Read the model definition and answer for the solid it produces. Units are mm, in the model's axes. Face numbers are marked on the shaded views. A direction names the side the tool comes from. Coordinates: 2 decimals unless noted, no trailing zeros. Write each loop counter-clockwise with the first axis right and the second up, starting at its lowest first coordinate (ties: lowest second). Pieces come first, ordered by that corner, then holes. Notation, with made-up numbers: (-8.75, -11.75) -> (18.25, -11.75) arc R20 ccw to (18.25, 10.25) -> close; hole circle Ø10 at (-30.5, 88.25). An arc over 180 degrees is marked (long way). Use CSV: the item, a comma, the result in double quotes.
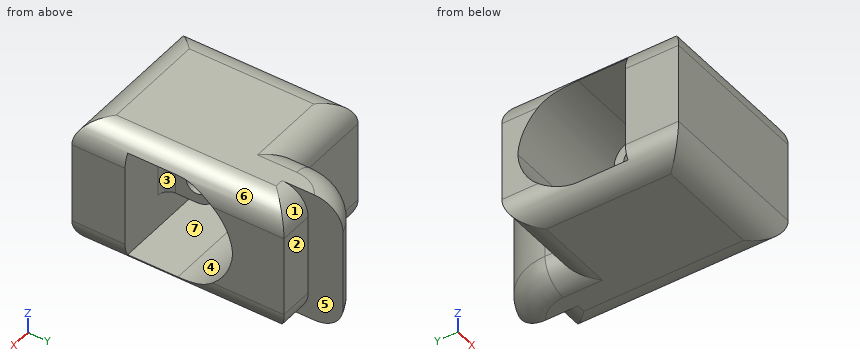
from build123d import *

# Parameters (mm, degrees)
BOSS_EXTRUDE1_DEPTH = 63.5
SKETCH3_W           = 103
SKETCH3_H           = 103
CUT_EXTRUDE1_DEPTH  = 211.692895559
BOSS_EXTRUDE2_DEPTH = 20
FILLET1_R           = 55
SKETCH6_R           = 10
CUT_EXTRUDE2_DEPTH  = 176.866755526
FILLET2_R           = 10
FILLET3_R           = 25


with BuildPart() as part:
    # Sketch2 → Boss-Extrude1 (new, symmetric)
    with BuildSketch(Plane.XY):
        with BuildLine():
            Line((-37.021158778, -102.394460884), (112.91726901, -102.394460884))
            Line((112.91726901, -102.394460884), (112.91726901, 63.318112544))
            Line((112.91726901, 63.318112544), (112.91726901, 100.457569387))
            Line((112.91726901, 100.457569387), (79.814777063, 100.457569387))
            Line((79.814777063, 100.457569387), (79.814777063, 133.707569387))
            ThreePointArc((79.814777063, 133.707569387), (50.885133933, 112.867809308), (39.821527553, 78.973614146))
            Line((39.821527553, 78.973614146), (39.821527553, 66.568112544))
            Line((39.821527553, 66.568112544), (-37.021158778, 66.568112544))
            Line((-37.021158778, 66.568112544), (-37.021158778, -102.394460884))
        make_face()
    extrude(amount=BOSS_EXTRUDE1_DEPTH, both=True)

    # Sketch3 → Cut-Extrude1 (cut, through all)
    with BuildSketch(Plane(origin=(112.91726901, 0, 0), x_dir=(0, 0, -1), z_dir=(1, 0, 0))):
        Rectangle(SKETCH3_W, SKETCH3_H)
    extrude(amount=-CUT_EXTRUDE1_DEPTH, mode=Mode.SUBTRACT)

    # Sketch5 → Boss-Extrude2 (add, symmetric)
    with BuildSketch(Plane.ZY.offset(-37.948055116)):
        with BuildLine():
            Line((19, -51.5), (-19, -51.5))
            Line((-19, -51.5), (-19, -21.5))
            ThreePointArc((-19, -21.5), (0, -2.5), (19, -21.5))
            Line((19, -21.5), (19, -51.5))
        make_face()
    extrude(amount=BOSS_EXTRUDE2_DEPTH, both=True)

    # Fillet1
    # the kernel refuses this fillet: 55 mm, written as the material it adds along each edge
    with BuildSketch(Plane(origin=(112.91726901, 51.5, 51.5), x_dir=(0, 0, -1), z_dir=(-1, 0, 0))) as fillet1_piece_1:
        with BuildLine():
            CenterArc((FILLET1_R, FILLET1_R), FILLET1_R, 180, 90)
            Line((0, FILLET1_R), (0, 0))
            Line((0, 0), (FILLET1_R, 0))
        make_face()
    extrude(amount=149.938427788)
    with BuildSketch(Plane(origin=(112.91726901, 51.5, -51.5), x_dir=(0, 0, 1), z_dir=(-1, 0, 0))) as fillet1_piece_2:
        with BuildLine():
            CenterArc((FILLET1_R, -FILLET1_R), FILLET1_R, 90, 90)
            Line((0, -FILLET1_R), (0, 0))
            Line((0, 0), (FILLET1_R, 0))
        make_face()
    extrude(amount=149.938427788)

    # Sketch6 → Cut-Extrude2 (cut, through all)
    with BuildSketch(Plane.ZY.offset(-17.948055116)):
        with Locations((0, -21.5)):
            Circle(SKETCH6_R)
    extrude(amount=-CUT_EXTRUDE2_DEPTH, mode=Mode.SUBTRACT)

    # Fillet2
    fillet2_edges = [part.edges().sort_by_distance(p)[0] for p in [
        (57.948055116, -51.5, 0),
        (17.948055116, -51.5, 0),
    ]]
    fillet(fillet2_edges, radius=FILLET2_R)

    # Fillet3
    # the kernel refuses this fillet: 25 mm, written as the material it takes off along each edge
    with BuildSketch(Plane(origin=(39.821527553, 78.973614146, -63.5), x_dir=(0, 0, 1), z_dir=(0, -1, 0)), Plane(origin=(39.821527553, 78.973614146, 63.5), x_dir=(1, 0, 0), z_dir=(0, -1, 0))) as fillet3_piece_1:
        with BuildLine():
            CenterArc((FILLET3_R, -FILLET3_R), FILLET3_R, 90, 90)
            Line((0, -FILLET3_R), (0, 0))
            Line((0, 0), (FILLET3_R, 0))
        make_face()
    extrude(amount=12.405501602, mode=Mode.SUBTRACT)
    with BuildSketch(Plane(origin=(97.272046317, 78.973614146, -63.5), x_dir=(0.7028717188946543, 0.711316629060557, 0), z_dir=(0.711316629060557, -0.7028717188946543, 0))) as fillet3_piece_2:
        with BuildLine():
            CenterArc((57.450518764 - FILLET3_R, FILLET3_R), FILLET3_R, 270, 90)
            Line((57.450518764 - FILLET3_R, 0), (57.450518764, 0))
            Line((57.450518764, 0), (57.450518764, FILLET3_R))
        make_face()
    revolve(axis=Axis((97.272046317, 78.973614146, -63.5), (0, 0, 1)), revolution_arc=134.657858898, mode=Mode.SUBTRACT)
    with BuildSketch(Plane(origin=(-99.521158778, -102.394460884, 63.5), x_dir=(0, 0, -1), z_dir=(1, 0, 0))) as fillet3_piece_3:
        with BuildLine():
            CenterArc((FILLET3_R, FILLET3_R), FILLET3_R, 180, 90)
            Line((0, FILLET3_R), (0, 0))
            Line((0, 0), (FILLET3_R, 0))
        make_face()
    extrude(amount=274.938427788, mode=Mode.SUBTRACT)
    with BuildSketch(Plane(origin=(97.272046317, 78.973614146, 63.5), x_dir=(0.7028717188946543, 0.711316629060557, 0), z_dir=(0.711316629060557, -0.7028717188946543, 0))) as fillet3_piece_4:
        with BuildLine():
            CenterArc((57.450518764 - FILLET3_R, -FILLET3_R), FILLET3_R, 0, 90)
            Line((57.450518764, -FILLET3_R), (57.450518764, 0))
            Line((57.450518764, 0), (57.450518764 - FILLET3_R, 0))
        make_face()
    revolve(axis=Axis((97.272046317, 78.973614146, 63.5), (0, 0, 1)), revolution_arc=134.657858898, mode=Mode.SUBTRACT)
    with BuildSketch(Plane(origin=(39.821527553, 66.568112544, 63.5), x_dir=(0, -1, 0), z_dir=(-1, 0, 0)), Plane(origin=(39.821527553, 66.568112544, -63.5), x_dir=(0, 0, 1), z_dir=(-1, 0, 0))) as fillet3_piece_5:
        with BuildLine():
            CenterArc((FILLET3_R, -FILLET3_R), FILLET3_R, 90, 90)
            Line((0, -FILLET3_R), (0, 0))
            Line((0, 0), (FILLET3_R, 0))
        make_face()
    extrude(amount=139.342686331, mode=Mode.SUBTRACT)
    with BuildSketch(Plane(origin=(-37.021158778, 129.068112544, 63.5), x_dir=(0, 0, -1), z_dir=(0, -1, 0))) as fillet3_piece_6:
        with BuildLine():
            CenterArc((FILLET3_R, FILLET3_R), FILLET3_R, 180, 90)
            Line((0, FILLET3_R), (0, 0))
            Line((0, 0), (FILLET3_R, 0))
        make_face()
    extrude(amount=293.962573428, mode=Mode.SUBTRACT)
    with BuildSketch(Plane(origin=(112.91726901, 162.957569387, 63.5), x_dir=(-1, 0, 0), z_dir=(0, -1, 0)), Plane(origin=(112.91726901, -164.894460884, -63.5), x_dir=(-1, 0, 0), z_dir=(0, 1, 0))) as fillet3_piece_7:
        with BuildLine():
            CenterArc((FILLET3_R, FILLET3_R), FILLET3_R, 180, 90)
            Line((0, FILLET3_R), (0, 0))
            Line((0, 0), (FILLET3_R, 0))
        make_face()
    extrude(amount=327.852030272, mode=Mode.SUBTRACT)
    with BuildSketch(Plane(origin=(-99.521158778, -102.394460884, -63.5), x_dir=(0, 0, 1), z_dir=(1, 0, 0))) as fillet3_piece_8:
        with BuildLine():
            CenterArc((FILLET3_R, -FILLET3_R), FILLET3_R, 90, 90)
            Line((0, -FILLET3_R), (0, 0))
            Line((0, 0), (FILLET3_R, 0))
        make_face()
    extrude(amount=274.938427788, mode=Mode.SUBTRACT)
    with BuildSketch(Plane(origin=(-37.021158778, 129.068112544, -63.5), x_dir=(0, 0, 1), z_dir=(0, -1, 0))) as fillet3_piece_9:
        with BuildLine():
            CenterArc((FILLET3_R, -FILLET3_R), FILLET3_R, 90, 90)
            Line((0, -FILLET3_R), (0, 0))
            Line((0, 0), (FILLET3_R, 0))
        make_face()
    extrude(amount=293.962573428, mode=Mode.SUBTRACT)
    with BuildSketch(Plane(origin=(175.41726901, 100.457569387, -63.5), x_dir=(0, 0, 1), z_dir=(-1, 0, 0)), Plane(origin=(175.41726901, 100.457569387, 63.5), x_dir=(0, -1, 0), z_dir=(-1, 0, 0))) as fillet3_piece_10:
        with BuildLine():
            CenterArc((FILLET3_R, -FILLET3_R), FILLET3_R, 90, 90)
            Line((0, -FILLET3_R), (0, 0))
            Line((0, 0), (FILLET3_R, 0))
        make_face()
    extrude(amount=95.602491947, mode=Mode.SUBTRACT)
    with BuildSketch(Plane(origin=(39.821527553, 78.973614146, -63.5), x_dir=(0, 0, 1), z_dir=(0, -1, 0))) as fillet3_piece_11a_section:
        with BuildLine():
            CenterArc((FILLET3_R, -FILLET3_R), FILLET3_R, 90, 90)
            Line((0, -FILLET3_R), (0, 0))
            Line((0, 0), (FILLET3_R, 0))
        make_face()
    fillet3_piece_11a = extrude(amount=74.905501602, mode=Mode.PRIVATE)
    fillet3_piece_11a = split(fillet3_piece_11a, bisect_by=Plane(origin=(45.48140541, 66.568112544, -57.840122143), z_dir=(0, -1, 0)), keep=Keep.TOP, mode=Mode.PRIVATE)
    with BuildSketch(Plane(origin=(102.321527553, 66.568112544, -63.5), x_dir=(0, 0, 1), z_dir=(-1, 0, 0))) as fillet3_piece_11b_section:
        with BuildLine():
            CenterArc((FILLET3_R, -FILLET3_R), FILLET3_R, 90, 90)
            Line((0, -FILLET3_R), (0, 0))
            Line((0, 0), (FILLET3_R, 0))
        make_face()
    fillet3_piece_11b = extrude(amount=201.842686331, mode=Mode.PRIVATE)
    fillet3_piece_11b = split(fillet3_piece_11b, bisect_by=Plane(origin=(39.821527553, 60.908234687, -57.840122143), z_dir=(1, 0, 0)), keep=Keep.TOP, mode=Mode.PRIVATE)
    fillet3_piece_11 = fillet3_piece_11a & fillet3_piece_11b
    add(fillet3_piece_11, mode=Mode.SUBTRACT)
    with BuildSketch(Plane(origin=(39.821527553, 78.973614146, 63.5), x_dir=(1, 0, 0), z_dir=(0, -1, 0))) as fillet3_piece_12a_section:
        with BuildLine():
            CenterArc((FILLET3_R, -FILLET3_R), FILLET3_R, 90, 90)
            Line((0, -FILLET3_R), (0, 0))
            Line((0, 0), (FILLET3_R, 0))
        make_face()
    fillet3_piece_12a = extrude(amount=74.905501602, mode=Mode.PRIVATE)
    fillet3_piece_12a = split(fillet3_piece_12a, bisect_by=Plane(origin=(45.48140541, 66.568112544, 57.840122143), z_dir=(0, -1, 0)), keep=Keep.TOP, mode=Mode.PRIVATE)
    with BuildSketch(Plane(origin=(102.321527553, 66.568112544, 63.5), x_dir=(0, -1, 0), z_dir=(-1, 0, 0))) as fillet3_piece_12b_section:
        with BuildLine():
            CenterArc((FILLET3_R, -FILLET3_R), FILLET3_R, 90, 90)
            Line((0, -FILLET3_R), (0, 0))
            Line((0, 0), (FILLET3_R, 0))
        make_face()
    fillet3_piece_12b = extrude(amount=201.842686331, mode=Mode.PRIVATE)
    fillet3_piece_12b = split(fillet3_piece_12b, bisect_by=Plane(origin=(39.821527553, 60.908234687, 57.840122143), z_dir=(1, 0, 0)), keep=Keep.TOP, mode=Mode.PRIVATE)
    fillet3_piece_12 = fillet3_piece_12a & fillet3_piece_12b
    add(fillet3_piece_12, mode=Mode.SUBTRACT)


solid = part.part
1. A tool of negligible diameter and unlimited length cuts with its end or side. For the marked faces 1, 2, 3 and 4, from which of +Z, -Z, +X, -X, +Y, -Y can it reach the whole face along a straight path? Write none if from no direction.
Solutions:
face 1,"+Z, +X, +Y"
face 2,"+Z, -Z, +X, +Y"
face 3,"+X"
face 4,"+X, -X"
2. Find the intervals of material crossed by line 1 along Y through (x, z) = (29, 0); line 2 along Z through (x, y) = (50, -21); line 3 along Z through (x, y) = (-2.5, -46), in increasing order.
Solutions:
line 1,"y = -102.39 to -31.5, -11.5 to -2.5, 51.39 to 66.57"
line 2,"z = -63.5 to -51.5, -18.99 to -9.99, 9.99 to 18.99, 51.5 to 63.5"
line 3,"z = -63.5 to -51.5, 51.5 to 63.5"
3. A cutting plane is placed at A-A (x = 99). Give the vertices of the cut face in (y, z), and give its area (3 significant figures).
Solutions:
outline,"(-102.39, -38.5) arc R25 ccw to (-88.48, -60.91) -> (86.54, -60.91) arc R25 ccw to (100.46, -38.5) -> (100.46, 38.5) arc R25 ccw to (86.54, 60.91) -> (-88.48, 60.91) arc R25 ccw to (-102.39, 38.5) -> close; hole (-51.5, -51.5) -> (-3.5, -51.5) arc R55 ccw to (51.39, 0) arc R55 ccw to (-3.5, 51.5) -> (-51.5, 51.5) -> close"
area,"15,000 mm^2"
4. A cutting plane is placed at C-C (y = -85.5). Give the vertices of the cut face in (x, z), and give its area (3 significant figures).
Solutions:
outline,"(-37.02, -38.5) arc R25 ccw to (-20.13, -62.15) -> (96.02, -62.15) arc R25 ccw to (112.92, -38.5) -> (112.92, 38.5) arc R25 ccw to (96.02, 62.15) -> (-20.13, 62.15) arc R25 ccw to (-37.02, 38.5) -> close"
area,"18,200 mm^2"
5. A cutting plane is placed at B-B (y = 36). Give the vertices of the cut face in (x, z), and give its area (3 significant figures).
Solutions:
outline,"(-37.02, -38.5) arc R25 ccw to (-12.02, -63.5) -> (87.92, -63.5) arc R25 ccw to (112.92, -38.5) -> (112.92, -34.77) -> (-37.02, -34.77) -> close; (-37.02, 34.77) -> (112.92, 34.77) -> (112.92, 38.5) arc R25 ccw to (87.92, 63.5) -> (-12.02, 63.5) arc R25 ccw to (-37.02, 38.5) -> close"
area,"8,080 mm^2"
6. Each of these flat-tipped pins is pushed along its axis until it touches: pin 1 Ø3.5 at (y, z) = (72, 9) entering from -X; pin 2 Ø3 at (x, z) = (21, 17) entering from +Y; pin 3 Ø8 at (x, z) = (-4, -49.5) entering from -Y. Where does it stop, or does it pass through?
Solutions:
pin 1,"stops at x = 39.82"
pin 2,"stops at y = 66.57"
pin 3,"stops at y = -101.39"
7. For a pull along Z with two mould halves and no side action, classify the marked faces 5, 6 and 7 as pulls with the +Z half, pulls with the -Z half, needs draft (parallel to the pull), parting line crosses it, or undercut.
Solutions:
face 5,"needs draft"
face 6,"pulls with the +Z half"
face 7,"undercut"
8. A cutting plane is placed at D-D (x = 43.5). Give the number of separate pieces and of enclosed holes in the cut face, and give its area (3 significant figures).
Solutions:
separate pieces,"1"
enclosed holes,"2"
area,"16,300 mm^2"
